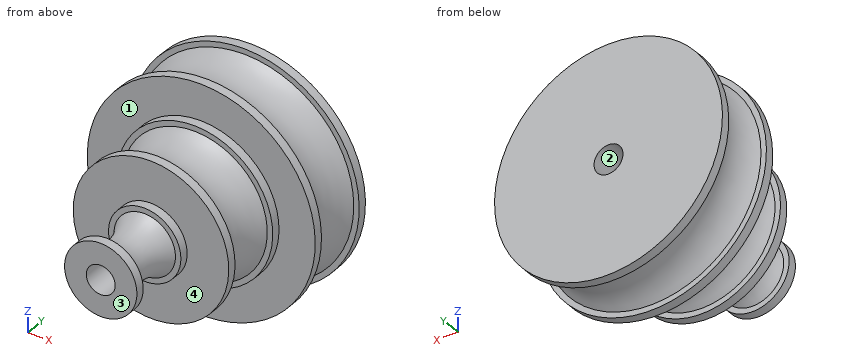
```python
from build123d import *


with BuildPart() as f1:
    # F0 (on Right) → F1 (revolve)
    with BuildSketch(Plane.YZ):
        Polygon((-15, 60), (-15, 8), (-10, 8), (-10, 63), (-15, 63), align=None)
        with BuildLine():
            Line((-45, 60), (-45, 8))
            Line((-45, 8), (-15, 8))
            Line((-15, 8), (-15, 60))
            ThreePointArc((-15, 60), (-30, 55.031032), (-45, 60))
        make_face()
        Polygon((-50, 8), (-45, 8), (-45, 60), (-45, 63), (-50, 63), (-50, 43), align=None)
        Polygon((-55, 8), (-50, 8), (-50, 43), (-55, 43), (-55, 40), align=None)
        with BuildLine():
            Line((-85, 8), (-55, 8))
            Line((-55, 8), (-55, 40))
            ThreePointArc((-55, 40), (-70, 35.031032), (-85, 40))
            Line((-85, 40), (-85, 8))
        make_face()
        Polygon((-90, 8), (-85, 8), (-85, 40), (-85, 43), (-90, 43), (-90, 20), align=None)
        Polygon((-95, 8), (-90, 8), (-90, 20), (-95, 20), (-95, 17), align=None)
        with BuildLine():
            Line((-125, 8), (-95, 8))
            Line((-95, 8), (-95, 17))
            ThreePointArc((-95, 17), (-110, 12.031032), (-125, 17))
            Line((-125, 17), (-125, 8))
        make_face()
        Polygon((-130, 8), (-125, 8), (-125, 17), (-125, 20), (-130, 20), align=None)
    revolve(axis=Axis((0, 30, 0), (0, -1, 0)))


solid = f1.part
```
The listing builds one solid part. Answer for the finished solid, in the listing's coordinates (mm). Face numbers are marked on the shaded views. A direction names the side the tool comes from. Round coordinates to 2 decimals unless told otherwise and drop trailing zeros. Write each loop counter-clockwise with the first axis right and the second up, starting at its lowest first coordinate (ties: lowest second). Pieces come first, ordered by that corner, then holes. Notation, with made-up numbers: (32, 53) -> (87, 53) arc R23 cw to (87, 79) -> close; hole circle Ø2 at (-8.5, 49). An arc over 180 degrees is marked (long way). Write item = value, one per line.
1) For a pull along X with two mould halves and no side action, classify the marked faces 1 and 2 as released by +X, released by -X, zero draft, split by the parting line, or undercut.
Check values:
face_1 = zero draft
face_2 = undercut
2) Section B-B on y = -82.5 is taken. Write down the section's boundary in (x, z).
Check values:
outline = circle Ø76.72 at (0, 0); hole circle Ø16 at (0, 0)
3) Straight lines are drawn through the part: line 1 along Z through (x, y) = (0, -86); line 2 along Y through (x, z) = (11, -40). For each, find the intervals that lie inside material, in ascending order. Write a range as [from, to].
Check values:
line_1 = [-43, -8], [8, 43]
line_2 = [-90, -85], [-55, -10]
4) Section A-A on y = -114.5 is taken. Write down the section's boundary in (x, z).
Check values:
outline = circle Ø24.87 at (0, 0); hole circle Ø16 at (0, 0)
5) Given pin 1 (8 mm diameter, centred on x = 7, y = -79, fed in from -Z); pin 2 (6 mm diameter, centred on y = -46.5, z = -19.5, fed in from -X); pin 3 (20 mm diameter, centred on x = 0, z = -3.5, fed in from +Y), each flat-ended and moving along its own axis, determine where each tip first touches the part or whether it passes through.
Check values:
pin_1 = -38.11
pin_2 = -60.8
pin_3 = -10
6) Which of the six approach directions +Z, -Z, +X, -X, +Y, -Y give full straight-line access (tool end or side, diameter ignored) to the marked faces 3 and 4?
Check values:
face_3 = +Z, -Z, +X, -X, -Y
face_4 = -Y
